Geometry: final body of the model. Coordinates: model frame, mm. A direction names the side the tool comes from. Round coordinates to 2 decimals unless told otherwise and drop trailing zeros. Write each loop counter-clockwise with the first axis right and the second up, starting at its lowest first coordinate (ties: lowest second). Pieces come first, ordered by that corner, then holes. Notation, with made-up numbers: (68.5, -13.5) -> (100.5, -13.5) arc R21 cw to (100.5, 10.5) -> close; hole circle Ø9 at (24, 61). An arc over 180 degrees is marked (long way). One line per item, written item: value. Start each with the question number.
from build123d import *

# Parameters (mm, degrees)
F0_R     = 7.9375
F0_R_2   = 11.828435
F0_R_3   = 12.7
F0_R_4   = 6.35
F1_DEPTH = 12.7
F2_DEPTH = 25.4
F3_DEPTH = 25.4


with BuildPart() as f1:
    # F0 (on Front) → F1 (new body)
    with BuildSketch(Plane.XZ):
        with BuildLine():
            Line((82.55, 7.45639), (82.55, 34.925))
            ThreePointArc((82.55, 34.925), (50.8, 66.675), (19.05, 34.925))
            Line((19.05, 34.925), (19.05, 33.3375))
            ThreePointArc((19.05, 33.3375), (17.655096, 29.969904), (14.2875, 28.575))
            Line((14.2875, 28.575), (-14.2875, 28.575))
            ThreePointArc((-14.2875, 28.575), (-17.655096, 29.969904), (-19.05, 33.3375))
            Line((-19.05, 33.3375), (-19.05, 34.925))
            ThreePointArc((-19.05, 34.925), (-50.8, 66.675), (-82.55, 34.925))
            Line((-82.55, 34.925), (-82.55, 7.45639))
            ThreePointArc((-82.55, 7.45639), (-83.623483, 4.44432), (-86.36, 2.790112))
            ThreePointArc((-86.36, 2.790112), (-101.503534, -17.789696), (-82.55, -34.925))
            Line((-82.55, -34.925), (-53.975, -34.925))
            ThreePointArc((-53.975, -34.925), (-47.239808, -37.714808), (-44.45, -44.45))
            Line((-44.45, -44.45), (-44.45, -51.575074))
            ThreePointArc((-44.45, -51.575074), (-41.660192, -58.310266), (-34.925, -61.100074))
            Line((-34.925, -61.100074), (-18.634955, -61.100074))
            Line((-18.634955, -61.100074), (-18.634955, -48.400074))
            ThreePointArc((-18.634955, -48.400074), (0.011654, -28.578944), (19.449271, -47.625))
            Line((19.449271, -47.625), (19.449271, -60.325))
            Line((19.449271, -60.325), (34.925, -60.325))
            ThreePointArc((34.925, -60.325), (41.660192, -57.535192), (44.45, -50.8))
            Line((44.45, -50.8), (44.45, -44.45))
            ThreePointArc((44.45, -44.45), (47.239808, -37.714808), (53.975, -34.925))
            Line((53.975, -34.925), (82.55, -34.925))
            ThreePointArc((82.55, -34.925), (101.503534, -17.789696), (86.36, 2.790112))
            ThreePointArc((86.36, 2.790112), (83.623483, 4.44432), (82.55, 7.45639))
        make_face()
        with Locations((-82.55, -15.875)):
            Circle(F0_R, mode=Mode.SUBTRACT)
        Circle(F0_R_2, mode=Mode.SUBTRACT)
        with Locations((82.55, -15.875)):
            Circle(F0_R, mode=Mode.SUBTRACT)
        with Locations((-50.8, 34.925)):
            Circle(F0_R_3, mode=Mode.SUBTRACT)
        with Locations((50.8, 34.925)):
            Circle(F0_R_3, mode=Mode.SUBTRACT)
        with Locations((-82.55, -15.875)):
            Circle(F0_R)
        with Locations((-82.55, -15.875)):
            Circle(F0_R_4, mode=Mode.SUBTRACT)
        with Locations((82.55, -15.875)):
            Circle(F0_R)
        with Locations((82.55, -15.875)):
            Circle(F0_R_4, mode=Mode.SUBTRACT)
    extrude(amount=F1_DEPTH)

    # F0 (on Front) → F2 (join)
    with BuildSketch(Plane.XZ):
        with Locations((82.55, -15.875)):
            Circle(F0_R)
        with Locations((82.55, -15.875)):
            Circle(F0_R_4, mode=Mode.SUBTRACT)
    extrude(amount=-F2_DEPTH)

    # F0 (on Front) → F3 (join)
    with BuildSketch(Plane.XZ):
        with Locations((-82.55, -15.875)):
            Circle(F0_R)
        with Locations((-82.55, -15.875)):
            Circle(F0_R_4, mode=Mode.SUBTRACT)
    extrude(amount=-F3_DEPTH)


solid = f1.part
(1) Set-up query: faces 1 (the face through (-44.45, -6, -48)), 2 (the face through (44.45, -6, -48)), 3 (the face through (0, -6, 28.575)). Return all of +Z, -Z, +X, -X, +Y, -Y with unobstructed straight access to the full face (end or side cutting, diameter ignored); none if empty.
(2) Section query D-D (z = 17). Output: boundary loops of the cut face in (x, y), and give its area (3 significant figures).
(3) Section query A-A (z = 0). Output: boundary loops of the cut face in (x, y), and give its area (3 significant figures).
(4) Pull-direction query (X, two-part tool) for faces 4 (the face through (-0.412, -6.261, -28.592)), 5 (the face through (83.65, -6.26, 4.41)), 6 (the face through (68, -6, -34.925)); classes: pulls with the +X half, pulls with the -X half, needs draft (parallel to the pull), parting line crosses it, or undercut.
(5) Section query C-C (y = 3). Count the separate pieces of the cut face and the enclosed holes in it, and give its area (3 significant figures).
(6) Pin query (flat end, axial travel): pin 1 (12 mm diameter, centred on x = -68.5, y = 1, fed in from +Z); pin 2 (5 mm diameter, centred on y = -7.5, z = -48, fed in from +X); pin 3 (1 mm diameter, centred on y = -4, z = 37.5, fed in from +X); pin 4 (16.5 mm diameter, centred on x = -82.55, z = -15.875, fed in from +Y). Return the tip coordinate at first contact, or that it passes through.
(7) Section query B-B (x = 50.8). Output: boundary loops of the cut face in (y, z) (3 decimals), and give its area (3 significant figures).
(8) Line query: probe 1 along X at (y, z) = (-10.5, 26.5); probe 2 along Z at (x, y) = (0, -5) (3 decimals); probe 3 along Y at (x, z) = (-14, 20.5). Output: solid intervals per line, ascending.
Results list:
1. face 1: -Z, -X, +Y, -Y
1. face 2: -Z, +X, +Y, -Y
1. face 3: +Z, +Y, -Y
2. outline: (-82.55, -12.7) -> (82.55, -12.7) -> (82.55, 0) -> (-82.55, 0) -> close
2. area: 2,100 mm^2
3. outline: (-93.08, -12.7) -> (-11.83, -12.7) -> (-11.83, 0) -> (-93.08, 0) -> close; (11.83, -12.7) -> (93.08, -12.7) -> (93.08, 0) -> (11.83, 0) -> close
3. area: 2,060 mm^2
4. face 4: undercut
4. face 5: pulls with the +X half
4. face 6: needs draft
5. separate pieces: 2
5. enclosed holes: 2
5. area: 143 mm^2
6. pin 1: stops at z = 64.41
6. pin 2: stops at x = 44.45
6. pin 3: stops at x = 82.48
6. pin 4: stops at y = 25.4
7. outline: (-12.7, -35.47) -> (0, -35.47) -> (0, 22.225) -> (-12.7, 22.225) -> close; (-12.7, 47.625) -> (0, 47.625) -> (0, 66.675) -> (-12.7, 66.675) -> close
7. area: 975 mm^2
8. probe 1: x = -82.55 to -60.3, -41.3 to 41.3, 60.3 to 82.55
8. probe 2: z = -28.579 to -11.828, 11.828 to 28.575
8. probe 3: y = -12.7 to 0
